Check sheet for the drawn part. Datum: minimum x, y, z corner. Units: mm. Give positions to 0.01 mm unless a question says otherwise; leave off trailing zeros. Loops run counter-clockwise (first coordinate to the right, second up) from the corner with the lowest first, then second, coordinate; pieces in that order, holes last. Notation, with made-up numbers: (56.5, 64) - (66.5, 64) arc R17 ccw to (66.5, 72) - close; hole circle Ø9 at (83, -24.5). An arc over 180 degrees is marked (long way). Use a Markdown table: item, result. Add a question column.
1. Cross-section at B-B on z = 15.5. Enter the section's corners in (x, y).
2. Depth check by flat-ended pin: P1, Ø1, axis at y = 1.5, z = 0.5, coming from the -X side; P2, Ø1, axis at y = 1, z = 1, coming from the +X side; P3, Ø0.6, axis at x = 25.5, y = 1.5, coming from the -Z side; P4, Ø4, axis at x = 28, z = 30.5, coming from the -Y side. Enter the tip coordinate at first touch or a pass-through.
3. Material ranges on L1, parallel to Z at x = 25, y = 1.1; L2, parallel to X at y = 1.9, z = 41, recorded low to high.
4. Cross-section at C-C on x = 37. Enter the section's corners in (y, z).
5. Cross-section at A-A on y = 1. Enter the section's corners in (x, z), and give its area (3 significant figures).
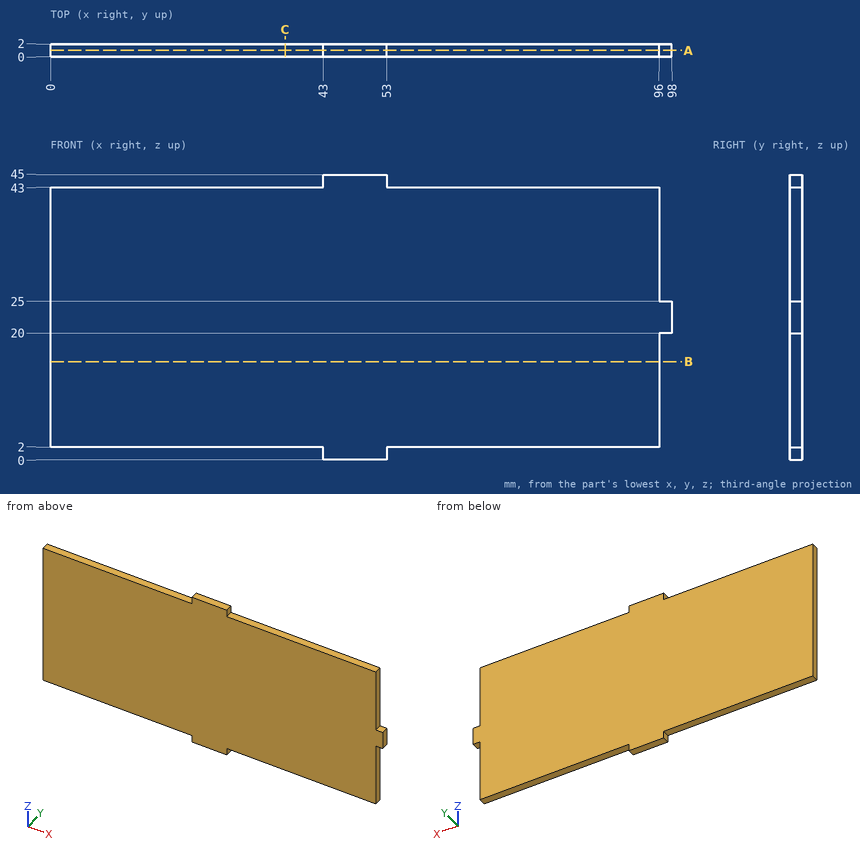
Values found:
| question | item | result |
|---|---|---|
| 1 | outline | (0, 0) - (96, 0) - (96, 2) - (0, 2) - close |
| 2 | P1 | stops at x = 43 |
| 2 | P2 | stops at x = 53 |
| 2 | P3 | stops at z = 2 |
| 2 | P4 | stops at y = 0 |
| 3 | L1 | z = 2 to 43 |
| 3 | L2 | x = 0 to 96 |
| 4 | outline | (0, 2) - (2, 2) - (2, 43) - (0, 43) - close |
| 5 | outline | (0, 2) - (43, 2) - (43, 0) - (53, 0) - (53, 2) - (96, 2) - (96, 20) - (98, 20) - (98, 25) - (96, 25) - (96, 43) - (53, 43) - (53, 45) - (43, 45) - (43, 43) - (0, 43) - close |
| 5 | area | 3,990 mm2 |
